Geometry check sheet. Reference: the model listing, model coordinates, mm. Face numbers are marked on the shaded views. A direction names the side the tool comes from. Give positions to 0.01 mm unless a question says otherwise; leave off trailing zeros. Write each loop counter-clockwise with the first axis right and the second up, starting at its lowest first coordinate (ties: lowest second). Pieces come first, ordered by that corner, then holes. Notation, with made-up numbers: (-34, 67) -> (-23, 67) arc R36 ccw to (-23, 105) -> close; hole circle Ø8 at (51.5, -22). An arc over 180 degrees is marked (long way). Write item = value, one per line. Start each with the question number.
1. Thickness scan on line 1 along Z through (x, y) = (9.5, 4.7); line 2 along Z through (x, y) = (5, 2.65); line 3 along Z through (x, y) = (24, 2.9). Record the ranges inside material, lowest first.
2. Cross-section at A-A, the plane x = 24.5. Record the cut outline in (y, z), plus the area to 3 significant figures.
3. Depth check by flat-ended pin: P1, Ø4, axis at x = 20.5, z = -56, coming from the +Y side; P2, Ø0.7, axis at x = 4, y = 2.5, coming from the -Z side; P3, Ø2, axis at x = 2, z = -34, coming from the +Y side; P4, Ø2.5, axis at x = 3, z = -61.8, coming from the +Y side. Enter the tip coordinate at first touch or a pass-through.
4. Set-up check for the marked faces 1, 2 and 3: record each of +Z, -Z, +X, -X, +Y, -Y from which the full face is reachable in a straight line by a thin tool's end or side.
5. Mould release check, pull along Z, two halves, no side actions. Record for the marked faces 4 and 5: pulls with the +Z half, pulls with the -Z half, needs draft (parallel to the pull), parting line crosses it, or undercut.
6. Cross-section at C-C, the plane z = -41.5. Record the cut outline in (x, y), plus the area to 3 significant figures.
7. Cross-section at B-B, the plane z = -48.5. Record the cut outline in (x, y).
Autodesk Fusion 360 part; units mm, degrees
sketch "Sketch1" plane through (0, 0, 0) normal (0, 1, 0) x (1, 0, 0)
  line L0 (0, 0) -> (32.4, 0)
  line L1 (32.4, 0) -> (32.4, 64.8)
  line L2 (32.4, 64.8) -> (0, 64.8)
  line L3 (0, 64.8) -> (0, 0)
  dimension "d1" = 64.8
  dimension "d2" = 32.4
extrude "Extrude1" add sketch "Sketch1" along normal blind 1.62
fillet "Fillet1" radius 2.6 4 edges at (0, 0.81, 0) (32.4, 0.81, 0) (0, 0.81, -64.8) (32.4, 0.81, -64.8)
sketch "Sketch2" plane through (0, 1.62, 0) normal (0, 1, 0) x (-1, 0, 0)
  circle A0 centre (-3, -3) radius 1.5
  circle A1 centre (-29.4, -3) radius 1.5
  circle A2 centre (-29.4, -61.8) radius 1.5
  circle A3 centre (-3, -61.8) radius 1.5
  line L0 (-29.8, -64.8) -> (-2.6, -64.8)
  line L1 (0, -62.2) -> (0, -2.6)
  line L2 (-32.4, -2.6) -> (-32.4, -62.2)
  line L3 (-2.6, 0) -> (-29.8, 0)
  dimension "d6" = 3
  dimension "d7" = 3
  dimension "d8" = 3
  dimension "d9" = 3
  dimension "d10" = 3
extrude "Extrude2" cut sketch "Sketch2" against normal blind 5
sketch "Sketch3" plane through (0, 0, 0) normal (0, -1, 0) x (1, 0, 0)
  line L0 (10.33, -57.1) -> (-0.77, -57.1)
  line L1 (-0.77, -57.1) -> (-0.77, -43.9)
  line L2 (-0.77, -43.9) -> (10.33, -43.9)
  line L3 (10.33, -43.9) -> (10.33, -57.1)
  line L4 (10.33, -21.2) -> (-0.77, -21.2)
  line L5 (-0.77, -21.2) -> (-0.77, -8)
  line L6 (-0.77, -8) -> (10.33, -8)
  line L7 (10.33, -8) -> (10.33, -21.2)
  line L8 (29.8, -64.8) -> (2.6, -64.8)
  line L9 (2.6, 0) -> (29.8, 0)
  line L10 (0, -62.2) -> (0, -2.6)
  dimension "d13" = 13.2
  dimension "d14" = 11.1
  dimension "d15" = 7.7
  dimension "d16" = 8
  dimension "d17" = 0.77
extrude "Extrude3" add sketch "Sketch3" against normal blind 5.73
sketch "Sketch4" plane through (0, 1.62, 0) normal (0, 1, 0) x (-1, 0, 0)
  line L0 (-22.2, -39.25) -> (-32.4, -39.25)
  line L1 (-32.4, -39.25) -> (-32.4, -49.6)
  line L2 (-32.4, -49.6) -> (-22.2, -49.6)
  line L3 (-22.2, -49.6) -> (-22.2, -39.25)
  line L4 (-29.8, -64.8) -> (-2.6, -64.8)
  point P0 (-32.4, -62.2)
  dimension "d20" = 10.35
  dimension "d21" = 10.2
  dimension "d22" = 15.2
extrude "Extrude4" add sketch "Sketch4" along normal blind 3.8
sketch "Sketch5" plane through (0, 1.62, 0) normal (0, 1, 0) x (-1, 0, 0)
  line L0 (-7.43, -37.16) -> (0.17, -37.16)
  line L1 (0.17, -37.16) -> (0.17, -28.16)
  line L2 (0.17, -28.16) -> (-7.43, -28.16)
  line L3 (-7.43, -28.16) -> (-7.43, -37.16)
  line L4 (0, -43.9) -> (0, -21.2)
  line L5 (-10.33, -43.9) -> (0, -43.9)
  dimension "d25" = 9
  dimension "d26" = 7.6
  dimension "d27" = 0.17
  dimension "d28" = 6.74
extrude "Extrude5" add sketch "Sketch5" along normal blind 3.2
fillet "Fillet2" radius 1 4 edges at (-0.085, 1.62, -28.16) (3.63, 4.82, -28.16) (3.63, 4.82, -37.16) (-0.085, 1.62, -37.16)
sketch "Sketch6" plane through (0, 1.62, 0) normal (0, 1, 0) x (-1, 0, 0)
  line L0 (-7.68, -4.38) -> (-12.18, -4.38)
  line L1 (-12.18, -4.38) -> (-12.18, -1.73)
  line L2 (-12.18, -1.73) -> (-7.68, -1.73)
  line L3 (-7.68, -1.73) -> (-7.68, -4.38)
  line L4 (-2.6, 0) -> (-29.8, 0)
  line L5 (0, -8) -> (0, -2.6)
  dimension "d32" = 4.5
  dimension "d33" = 2.65
  dimension "d34" = 1.73
  dimension "d35" = 7.68
extrude "Extrude6" add sketch "Sketch6" along normal blind 3.5
sketch "Sketch7" plane through (0, 0, -1.73) normal (0, 0, 1) x (1, 0, 0)
  circle A0 centre (9.93, 3.31) radius 0.95
  line L0 (7.68, 5.12) -> (12.18, 5.12)
  point P0 (9.93, 5.12)
  dimension "d38" = 1.9
  dimension "d39" = 1.81
extrude "Extrude7" add sketch "Sketch7" along normal blind 0.86
sketch "Sketch8" plane through (0, 1.62, 0) normal (0, 1, 0) x (-1, 0, 0)
  line L0 (-17.54, -6.8) -> (-25.14, -6.8)
  line L1 (-25.14, -6.8) -> (-25.14, -1)
  line L2 (-25.14, -1) -> (-17.54, -1)
  line L3 (-17.54, -1) -> (-17.54, -6.8)
  line L4 (-2.6, 0) -> (-29.8, 0)
  line L5 (-32.4, -2.6) -> (-32.4, -39.25)
  dimension "d42" = 5.8
  dimension "d43" = 7.6
  dimension "d44" = 1
  dimension "d45" = 7.26
extrude "Extrude8" add sketch "Sketch8" along normal blind 2.42
equation "d7 = 1.5 mm + d6 / 2"
equation "d8 = d7"
equation "d9 = d7"
equation "d10 = d7"
equation "d18 = -1 * ( 4.11 mm + 1.62 mm )"
equation "d39 = 0.86 mm + d38 / 2"
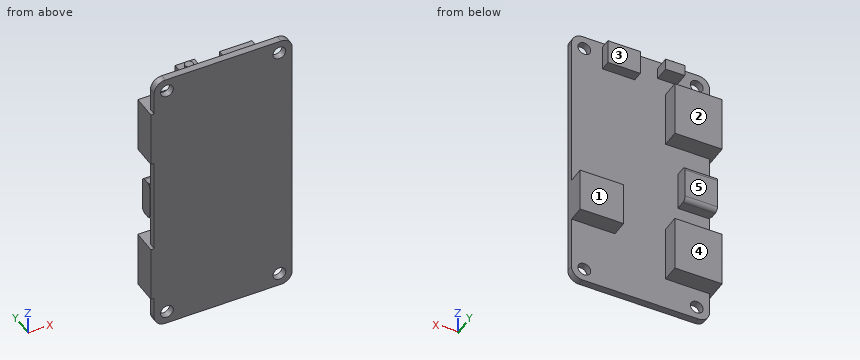
Answers:
q1.line_1 = -57.1 to -43.9, -21.2 to -8, -4.38 to -1.73
q1.line_2 = -57.1 to -43.9, -37.16 to -28.16, -21.2 to -8
q1.line_3 = -49.6 to -39.25, -6.8 to -1
q2.outline = (0, -64.8) -> (1.62, -64.8) -> (1.62, -49.6) -> (5.42, -49.6) -> (5.42, -39.25) -> (1.62, -39.25) -> (1.62, -6.8) -> (4.04, -6.8) -> (4.04, -1) -> (1.62, -1) -> (1.62, 0) -> (0, 0) -> close
q2.area = 158 mm^2
q3.P1 = 1.62
q3.P2 = -57.1
q3.P3 = 4.82
q3.P4 = through
q4.face_1 = +Z, -Z, +X, +Y
q4.face_2 = +Z, -Z, +X, -X, +Y
q4.face_3 = +Z, +X, +Y
q5.face_4 = needs draft
q5.face_5 = undercut
q6.outline = (0, 0) -> (32.4, 0) -> (32.4, 5.42) -> (22.2, 5.42) -> (22.2, 1.62) -> (0, 1.62) -> close
q6.area = 91.2 mm^2
q7.outline = (-0.77, 0) -> (32.4, 0) -> (32.4, 5.42) -> (22.2, 5.42) -> (22.2, 1.62) -> (10.33, 1.62) -> (10.33, 5.73) -> (-0.77, 5.73) -> close
